Input: dimensioned drawing with shaded views. Units: mm. Origin: part minimum x, y, z. A direction names the side the tool comes from. Round coordinates to 2 decimals unless told otherwise and drop trailing zeros. Loops run counter-clockwise (first coordinate to the right, second up) from the corner with the lowest first, then second, coordinate; pieces in that order, holes last. Notation, with made-up numbers: M 6,51 L 43,51 A29 ccw 43,89 Z; hole C 48.5,32 d10. An arc over 180 degrees is marked long. One line per item, written item: value.
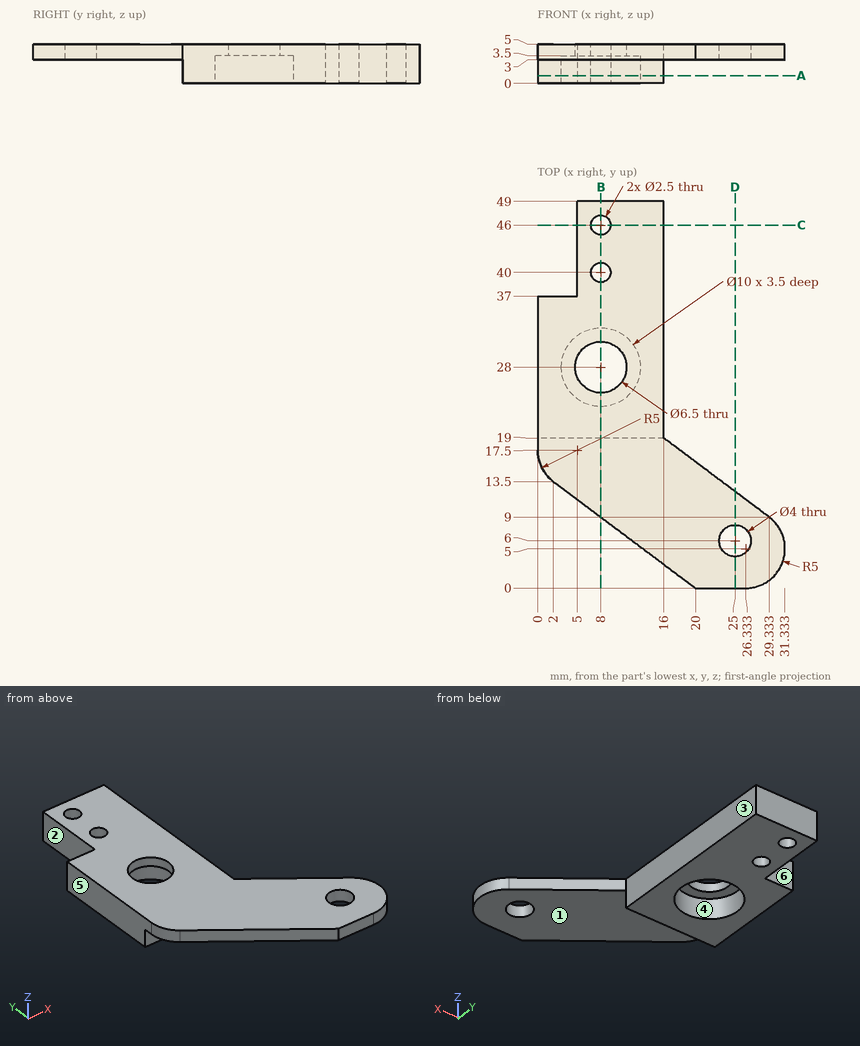
1. Pull-direction query (Y, two-part tool) for the marked faces 4, 5 and 6; classes: released by +Y, released by -Y, zero draft, split by the parting line, or undercut.
Report:
face 4: undercut
face 5: zero draft
face 6: released by +Y
2. Pin query (flat end, axial travel): pin 1 (3 mm diameter, centred on y = 10, z = 3.5, fed in from +X) (1 decimal); pin 2 (1.5 mm diameter, centred on x = 4, z = 1.5, fed in from +Y); pin 3 (4.5 mm diameter, centred on x = 25, y = 6, fed in from -Z). Return the tip coordinate at first contact, or that it passes through.
Report:
pin 1: stops at x = 29.9
pin 2: stops at y = 37
pin 3: stops at z = 3
3. Reachability of the marked faces 1, 2 and 3 from +Z, -Z, +X, -X, +Y, -Y: full face, straight path, thin tool, end or side. Return the list, or none.
Report:
face 1: -Z, +X, -X, -Y
face 2: +Z, -Z, -X, +Y
face 3: +Z, -Z, +X, +Y
4. Section query B-B (x = 8). Return the cut outline in (y, z).
Report:
outline: M 9,3 L 19,3 L 19,0 L 23,0 L 23,3.5 L 24.75,3.5 L 24.75,5 L 9,5 Z; M 31.25,3.5 L 33,3.5 L 33,0 L 38.75,0 L 38.75,5 L 31.25,5 Z; M 41.25,0 L 44.75,0 L 44.75,5 L 41.25,5 Z; M 47.25,0 L 49,0 L 49,5 L 47.25,5 Z
5. Ray query, line 1 (Y direction, x = 8, z = 1.75); line 2 (Z direction, x = 17.5, y = 7); line 3 (Y direction, x = 9, z = 3.95). Return the intervals inside material, ascending. Write a range as [from, to].
Report:
line 1: y = [19, 23], [33, 38.75], [41.25, 44.75], [47.25, 49]
line 2: z = [3, 5]
line 3: y = [8.25, 24.91], [31.09, 39.25], [40.75, 45.25], [46.75, 49]
6. Section query C-C (y = 46). Return the cut outline in (x, z), and give its area (3 significant figures).
Report:
outline: M 5,0 L 6.75,0 L 6.75,5 L 5,5 Z; M 9.25,0 L 16,0 L 16,5 L 9.25,5 Z
area: 42.5 mm2
7. Section query A-A (z = 1). Return the cut outline in (x, y).
Report:
outline: M 0,19 L 16,19 L 16,49 L 5,49 L 5,37 L 0,37 Z; hole C 8,28 d10; hole C 8,40 d2.5; hole C 8,46 d2.5
8. Section query D-D (x = 25). Return the cut outline in (y, z).
Report:
outline: M 0,3 L 4,3 L 4,5 L 0,5 Z; M 8,3 L 12.25,3 L 12.25,5 L 8,5 Z
